Read the model definition and answer for the solid it produces. Units are mm, in the model's axes. Face numbers are marked on the shaded views. A direction names the side the tool comes from. Round coordinates to 2 decimals unless told otherwise and drop trailing zeros. Loops run counter-clockwise (first coordinate to the right, second up) from the corner with the lowest first, then second, coordinate; pieces in that order, holes last. Notation, with made-up numbers: (75.5, -28.5) - (99.5, -28.5) arc R19 cw to (99.5, -2.5) - close; hole circle Ø3 at (31.5, 76.25). An arc over 180 degrees is marked (long way). Answer as CSV lines item,"result".
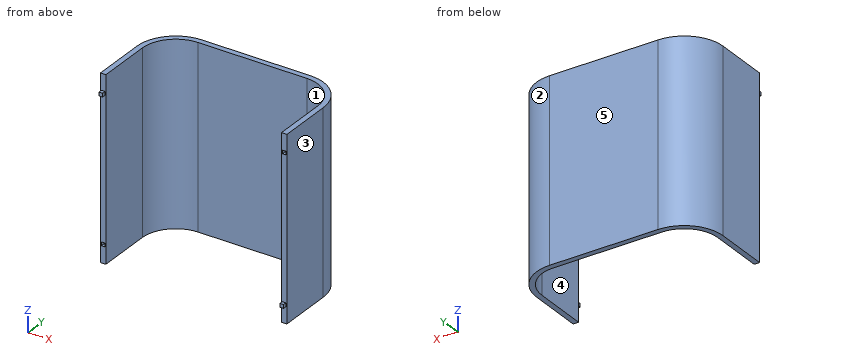
```python
from build123d import *

# Parameters (mm, degrees)
SKETCH2_W           = 15
SKETCH2_H           = 500
SKETCH3_W           = 10
SKETCH3_H           = 10
BOSS_EXTRUDE1_DEPTH = 10
SKETCH3_3_W         = 10
SKETCH3_3_H         = 10
CUT_EXTRUDE1_DEPTH  = 10


with BuildPart() as part:
    # Sweep1: sweep along a path in Sketch1
    with BuildLine(Plane.XY) as sweep1_path:
        Line((-250, 0), (-250, 150))
        ThreePointArc((-250, 150), (-220.710678119, 220.710678119), (-150, 250))
        Line((-150, 250), (150, 250))
        ThreePointArc((150, 250), (220.710678119, 220.710678119), (250, 150))
        Line((250, 150), (250, 0))
    # Sketch2 → Sweep1 (sweep)
    with BuildSketch(Plane(origin=(0, 0, 0), x_dir=(1, 0, 0), z_dir=(0, 1, 0))):
        with Locations((-250, 0)):
            Rectangle(SKETCH2_W, SKETCH2_H)
    sweep(path=sweep1_path.line)

    # Sketch3 → Boss-Extrude1 (add)
    with BuildSketch(Plane.XZ):
        with Locations((-250, 200)):
            Rectangle(SKETCH3_W, SKETCH3_H)
        with Locations((250, -200)):
            Rectangle(SKETCH3_W, SKETCH3_H)
    extrude(amount=BOSS_EXTRUDE1_DEPTH)

    # Sketch3<3> → Cut-Extrude1 (cut)
    with BuildSketch(Plane.XZ):
        with Locations((-250, -200)):
            Rectangle(SKETCH3_3_W, SKETCH3_3_H)
        with Locations((250, 200)):
            Rectangle(SKETCH3_3_W, SKETCH3_3_H)
    extrude(amount=-CUT_EXTRUDE1_DEPTH, mode=Mode.SUBTRACT)


solid = part.part
```
1) A cutting plane is placed at A-A, the plane y = 132. Determine the outline of the cut face in (x, z).
Entries:
outline,"(-257.5, -250) - (-242.5, -250) - (-242.5, 250) - (-257.5, 250) - close; (242.5, -250) - (257.5, -250) - (257.5, 250) - (242.5, 250) - close"
2) A cutting plane is placed at D-D, the plane x = -19. Determine the outline of the cut face in (y, z), plus the area to 3 significant figures.
Entries:
outline,"(242.5, -250) - (257.5, -250) - (257.5, 250) - (242.5, 250) - close"
area,"7,500 mm^2"
3) A cutting plane is placed at B-B, the plane z = 70.5. Determine the outline of the cut face in (x, y), plus the area to 3 significant figures.
Entries:
outline,"(-257.5, 0) - (-242.5, 0) - (-242.5, 150) arc R92.5 cw to (-150, 242.5) - (150, 242.5) arc R92.5 cw to (242.5, 150) - (242.5, 0) - (257.5, 0) - (257.5, 150) arc R107.5 ccw to (150, 257.5) - (-150, 257.5) arc R107.5 ccw to (-257.5, 150) - close"
area,"13,700 mm^2"
4) A cutting plane is placed at C-C, the plane y = 174.5. Determine the outline of the cut face in (x, z), plus the area to 3 significant figures.
Entries:
outline,"(-254.67, -250) - (-239.2, -250) - (-239.2, 250) - (-254.67, 250) - close; (239.2, -250) - (254.67, -250) - (254.67, 250) - (239.2, 250) - close"
area,"15,500 mm^2"
5) Find the intervals of material crossed by line 1 (X direction, y = 144, z = -49.5); line 2 (Y direction, x = 84, z = -63.5); line 3 (X direction, y = 219.5, z = -83), in increasing order.
Entries:
line 1,"x = -257.5 to -242.5, 242.5 to 257.5"
line 2,"y = 242.5 to 257.5"
line 3,"x = -232.01 to -211.04, 211.04 to 232.01"
6) Each of these flat-tipped pins is pushed along its axis until it touches: P1, Ø5, axis at y = -6, z = 202, coming from the +X side; P2, Ø16.5, axis at x = 250, z = 59, coming from the -Y side; P3, Ø3, axis at x = 249.5, z = 198.5, coming from the -Y side. Where does it stop, or does it pass through?
Entries:
P1,"stops at x = -245"
P2,"stops at y = 0"
P3,"stops at y = 10"
7) A tool of negligible diameter and unlimited length cuts with its end or side. For the marked faces 1 and 2, from which of +Z, -Z, +X, -X, +Y, -Y can it reach the whole face along a straight path? Write none if from no direction.
Entries:
face 1,"+Z, -Z, -Y"
face 2,"+Z, -Z, +X, +Y"
8) The mould has two halves that part along X. Classify the marked faces 3, 4 and 5: pulls with the +X half, pulls with the -X half, needs draft (parallel to the pull), parting line crosses it, or undercut.
Entries:
face 3,"pulls with the +X half"
face 4,"undercut"
face 5,"needs draft"
